from build123d import *

# Parameters (mm, degrees)
BOSS_EXTRUDE2_DEPTH = 100
SHELL2_T            = -2
SKETCH5_R           = 8
CUT_EXTRUDE1_DEPTH  = 100


with BuildPart() as part:
    # Sketch3 → Boss-Extrude2 (new body)
    with BuildSketch(Plane(origin=(0, 0, 0), x_dir=(1, 0, 0), z_dir=(0, 1, 0))):
        with BuildLine():
            Line((184.402855292, 224.204318802), (89.402855292, 224.204318802))
            Line((89.402855292, 224.204318802), (-5.597144708, 224.204318802))
            ThreePointArc((-5.597144708, 224.204318802), (-9.132678614, 222.739852708), (-10.597144708, 219.204318802))
            Line((-10.597144708, 219.204318802), (-10.597144708, -20.795681198))
            ThreePointArc((-10.597144708, -20.795681198), (-9.132678614, -24.331215104), (-5.597144708, -25.795681198))
            Line((-5.597144708, -25.795681198), (89.402855292, -25.795681198))
            Line((89.402855292, -25.795681198), (184.402855292, -25.795681198))
            ThreePointArc((184.402855292, -25.795681198), (187.938389198, -24.331215104), (189.402855292, -20.795681198))
            Line((189.402855292, -20.795681198), (189.402855292, 219.204318802))
            ThreePointArc((189.402855292, 219.204318802), (187.938389198, 222.739852708), (184.402855292, 224.204318802))
        make_face()
    extrude(amount=BOSS_EXTRUDE2_DEPTH)

    # Shell2
    shell2_openings = [part.faces().sort_by_distance(p)[0] for p in [
        (89.402855292, 100, -99.204318802),
    ]]
    offset(amount=SHELL2_T, openings=shell2_openings, kind=Kind.INTERSECTION)

    # Sketch5 → Cut-Extrude1 (cut)
    with BuildSketch(Plane.XY.offset(25.795681198)):
        with Locations((76.402855292, 50)):
            Circle(SKETCH5_R)
        with Locations((102.402855292, 50)):
            Circle(SKETCH5_R)
    extrude(amount=-CUT_EXTRUDE1_DEPTH, mode=Mode.SUBTRACT)


solid = part.part
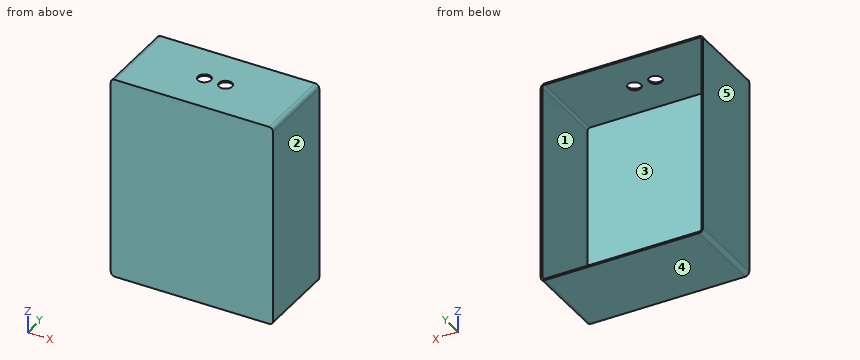
Verification items for the finished model (mm, model axes). Face numbers are marked on the shaded views. A direction names the side the tool comes from. Round coordinates to 2 decimals unless told otherwise and drop trailing zeros. Loops run counter-clockwise (first coordinate to the right, second up) from the corner with the lowest first, then second, coordinate; pieces in that order, holes last. Notation, with made-up numbers: (42, 38) - (58, 38) arc R29 cw to (58, 68) - close; hole circle Ø8 at (22.5, 53.25). An arc over 180 degrees is marked (long way). Answer in a Markdown table with one row per item. Add a question column.
Q1. Tool access check on the marked faces 1 and 2. Record the directions out of +Z, -Z, +X, -X, +Y, -Y that give a thin tool (end or side, any length) a straight path to the whole face; none if there is none.
Q2. Section check B-B on z = -174. Enter the section's corners in (x, y).
Q3. Release check for a two-part mould opening along Z. For the marked faces 3, 4 and 5 record: pulls with the +Z half, pulls with the -Z half, needs draft (parallel to the pull), parting line crosses it, or undercut.
Q4. Section check A-A on y = 50. Enter the section's corners in (x, z), plus the area to 3 significant figures.
Q5. Material ranges on line 1 (X direction, y = 75, z = -155); line 2 (Z direction, x = 122, y = 39.5); line 3 (Y direction, x = 67, z = -159.5), recorded low to high.
Q6. Gauge pin test, flat end, axial feed: pin 1 (1.5 mm diameter, centred on x = 82, z = -110.5, fed in from +Y). Record the tip position at first contact, or that the pin passes through.
Q7. Section check D-D on x = 126. Enter the section's corners in (y, z).
Q8. Section check C-C on y = 80. Enter the section's corners in (x, z), plus the area to 3 significant figures.
Found:
| question | item | result |
|---|---|---|
| 1 | face 1 | +Y |
| 1 | face 2 | +Z, -Z, +X, +Y, -Y |
| 2 | outline | (-10.6, 0) - (189.4, 0) - (189.4, 100) - (187.4, 100) - (187.4, 2) - (-8.6, 2) - (-8.6, 100) - (-10.6, 100) - close |
| 3 | face 3 | undercut |
| 3 | face 4 | pulls with the -Z half |
| 3 | face 5 | needs draft |
| 4 | outline | (-10.6, -219.2) arc R5 ccw to (-5.6, -224.2) - (184.4, -224.2) arc R5 ccw to (189.4, -219.2) - (189.4, 20.8) arc R5 ccw to (184.4, 25.8) - (110.4, 25.8) - (110.4, 23.8) - (184.4, 23.8) arc R3 cw to (187.4, 20.8) - (187.4, -219.2) arc R3 cw to (184.4, -222.2) - (-5.6, -222.2) arc R3 cw to (-8.6, -219.2) - (-8.6, 20.8) arc R3 cw to (-5.6, 23.8) - (68.4, 23.8) - (68.4, 25.8) - (-5.6, 25.8) arc R5 ccw to (-10.6, 20.8) - close; (84.4, 23.8) - (94.4, 23.8) - (94.4, 25.8) - (84.4, 25.8) - close |
| 4 | area | 1,710 mm² |
| 5 | line 1 | x = -10.6 to -8.6, 187.4 to 189.4 |
| 5 | line 2 | z = -224.2 to -222.2, 23.8 to 25.8 |
| 5 | line 3 | y = 0 to 2 |
| 6 | pin 1 | stops at y = 2 |
| 7 | outline | (0, -224.2) - (100, -224.2) - (100, -222.2) - (2, -222.2) - (2, 23.8) - (100, 23.8) - (100, 25.8) - (0, 25.8) - close |
| 8 | outline | (-10.6, -219.2) arc R5 ccw to (-5.6, -224.2) - (184.4, -224.2) arc R5 ccw to (189.4, -219.2) - (189.4, 20.8) arc R5 ccw to (184.4, 25.8) - (-5.6, 25.8) arc R5 ccw to (-10.6, 20.8) - close; hole (-8.6, -219.2) arc R3 ccw to (-5.6, -222.2) - (184.4, -222.2) arc R3 ccw to (187.4, -219.2) - (187.4, 20.8) arc R3 ccw to (184.4, 23.8) - (-5.6, 23.8) arc R3 ccw to (-8.6, 20.8) - close |
| 8 | area | 1,770 mm² |
